Verification items for this drawing (mm, ordinates from the low corner). A direction names the side the tool comes from. Round coordinates to 2 decimals unless told otherwise and drop trailing zeros. Order: outer loops, then holes, each group sorted by start corner. A loop starts at its lowest first (then second) coordinate and runs counter-clockwise, first axis right, second up. Notation, with made-up numbers: (36.25, 33) - (57.25, 33) arc R20 cw to (57.25, 68) - close; hole circle Ø2 at (34, -11). An arc over 180 degrees is marked (long way). One line per question, with ' | ' between items. Start each with the question number.
Q1. Tool access check on the marked faces 1 and 2. Record the directions out of +Z, -Z, +X, -X, +Y, -Y that give a thin tool (end or side, any length) a straight path to the whole face; none if there is none.
Q2. Gauge pin test, flat ends, axial feed: P1, Ø22, axis at x = 20, y = 146, coming from the +Z side; P2, Ø6, axis at y = 180, z = 15, coming from the -X side. Record the tip position at first contact, or that the pin passes through.
Q3. Sectioned sample at A-A, the plane z = 15. Enter the section's corners in (x, y), then the cut area to 3 significant figures.
Q4. Sectioned sample at B-B, the plane y = 180. Enter the section's corners in (x, z).
Q5. Sectioned sample at D-D, the plane x = 44.5. Enter the section's corners in (y, z).
Q6. Material ranges on line 1 along X through (y, z) = (108.5, 40.5); line 2 along Z through (x, y) = (48.7, 180); line 3 along Z through (x, y) = (21, 128.5), recorded low to high.
Q7. Mould release check, pull along X, two halves, no side actions. Record for the marked faces 3, 4 and 5: +X half, -X half, draft (parallel to the pull), parting line (faces both ways), or undercut.
Q8. Sectioned sample at C-C, the plane z = 30. Enter the section's corners in (x, y), then the cut area to 3 significant figures.
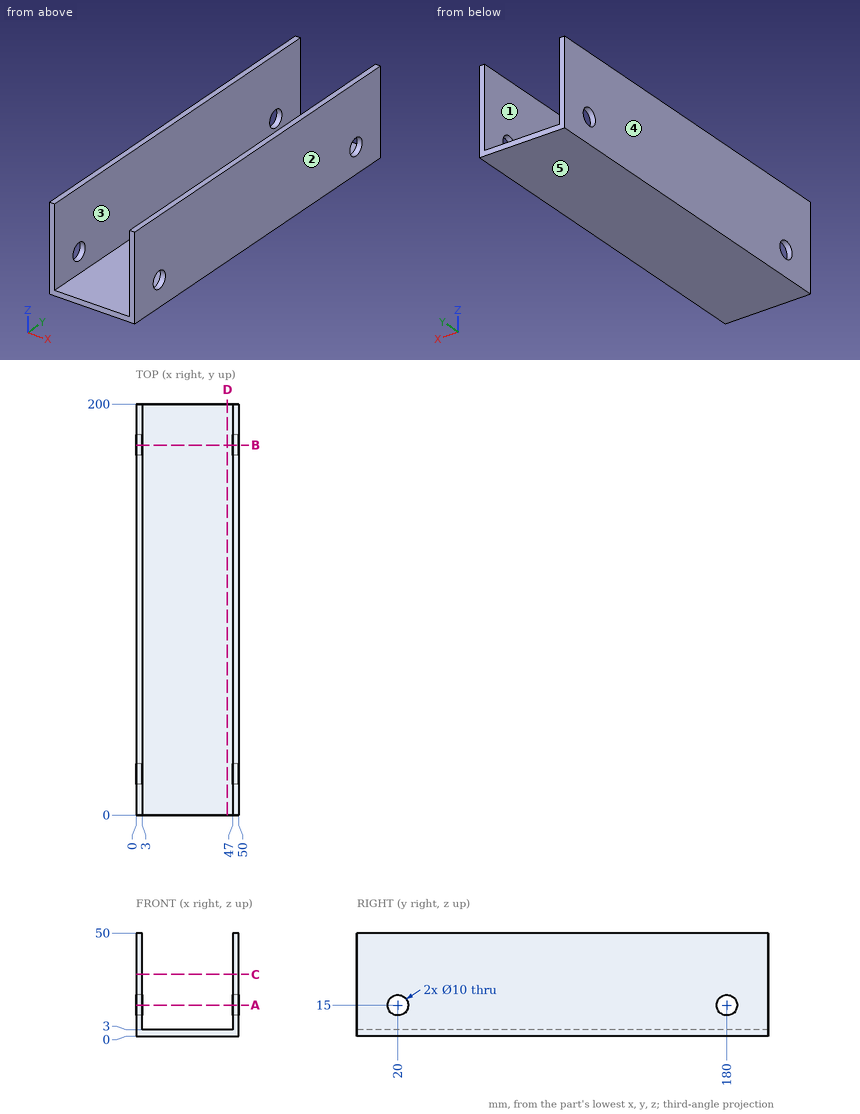
Determined:
1) face 1: +Z, +Y, -Y | face 2: +Z, -Z, +X, +Y, -Y
2) P1: stops at z = 3 | P2: passes through
3) outline: (0, 0) - (3, 0) - (3, 15) - (0, 15) - close; (0, 25) - (3, 25) - (3, 175) - (0, 175) - close; (0, 185) - (3, 185) - (3, 200) - (0, 200) - close; (47, 0) - (50, 0) - (50, 15) - (47, 15) - close; (47, 25) - (50, 25) - (50, 175) - (47, 175) - close; (47, 185) - (50, 185) - (50, 200) - (47, 200) - close | area: 1,080 mm2
4) outline: (0, 0) - (50, 0) - (50, 10) - (47, 10) - (47, 3) - (3, 3) - (3, 10) - (0, 10) - close; (0, 20) - (3, 20) - (3, 50) - (0, 50) - close; (47, 20) - (50, 20) - (50, 50) - (47, 50) - close
5) outline: (0, 0) - (200, 0) - (200, 3) - (0, 3) - close
6) line 1: x = 0 to 3, 47 to 50 | line 2: z = 0 to 10, 20 to 50 | line 3: z = 0 to 3
7) face 3: undercut | face 4: -X half | face 5: draft
8) outline: (0, 0) - (3, 0) - (3, 200) - (0, 200) - close; (47, 0) - (50, 0) - (50, 200) - (47, 200) - close | area: 1,200 mm2
